Part model, mm, in its own coordinate system. A direction names the side the tool comes from. Give positions to 0.01 mm unless a question says otherwise; leave off trailing zeros. Order: outer loops, then holes, each group sorted by start corner. A loop starts at its lowest first (then second) coordinate and runs counter-clockwise, first axis right, second up. Notation, with made-up numbers: M 52.25,44.5 L 98.25,44.5 A23 cw 98.25,67.5 Z; hole C 40.25,26 d6. An arc over 180 degrees is marked long. One line per question, with ' | ' between items.
```python
from build123d import *

# Parameters (mm, degrees)
SKETCH_1_R          = 1.5
EXTRUDE_1_DEPTH     = 3.3
CUT_EXTRUDE_1_DEPTH = 3.3


with BuildPart() as part:
    # Эскиз1 → Бобышка-Вытянуть1 (new body)
    with BuildSketch(Plane(origin=(0, 0, 0), x_dir=(1, 0, 0), z_dir=(0, 1, 0))):
        Polygon((0, 0), (0, 125), (-14, 125), (-14, 14), (-68, 14), (-68, 0), align=None)
        with Locations((-30, 4)):
            Circle(SKETCH_1_R, mode=Mode.SUBTRACT)
    extrude(amount=EXTRUDE_1_DEPTH)

    # Эскиз2 → Вырез-Вытянуть1 (cut)
    with BuildSketch(Plane(origin=(0, 3.3, 0), x_dir=(1, 0, 0), z_dir=(0, 1, 0))):
        Polygon((-15.4, 14), (-14.339339828, 12.939339828), (-12.939339828, 14.339339828), (-14, 15.4), align=None)
    extrude(amount=-CUT_EXTRUDE_1_DEPTH, mode=Mode.SUBTRACT)


solid = part.part
```
1. Mould opens along Z. For faces 3 (the flat face through (-34, 2, 0)), 4 (the flat face through (-11, 3.3, -49)), 5 (the cylindrical face through (-31.5, 1.63, -4.07)) say: released by +Z, released by -Z, zero draft, split by the parting line, or undercut.
Worked out:
face 3: released by +Z | face 4: zero draft | face 5: undercut
2. Slice it at C-C on z = -4. Give the cut face in (x, y).
Worked out:
outline: M -68,0 L -31.5,0 L -31.5,3.3 L -68,3.3 Z; M -28.5,0 L 0,0 L 0,3.3 L -28.5,3.3 Z
3. Slice it at A-A on y = 1.6. Give the cut face in (x, z).
Worked out:
outline: M -68,-14 L -15.4,-14 L -14.34,-12.94 L -12.94,-14.34 L -14,-15.4 L -14,-125 L 0,-125 L 0,0 L -68,0 Z; hole C -30,-4 d3
4. Slice it at B-B on x = -30. Give the cut face in (y, z), then the cut area to 3 significant figures.
Worked out:
outline: M 0,-14 L 3.3,-14 L 3.3,-5.5 L 0,-5.5 Z; M 0,-2.5 L 3.3,-2.5 L 3.3,0 L 0,0 Z | area: 36.3 mm2
5. Slice it at D-D on z = -29.5. Give the cut face in (x, y).
Worked out:
outline: M -14,0 L 0,0 L 0,3.3 L -14,3.3 Z
6. Probe L1, parallel to X at y = 2.55, z = -4; L2, parallel to Z at x = -30, y = 1.1; L3, parallel to X at y = 1.7, z = -27. List the from-to ranges inside material, lowest first. Write a range as from..to.
Worked out:
L1: x = -68..-31.5, -28.5..0 | L2: z = -14..-5.5, -2.5..0 | L3: x = -14..0
7. Tool access for faces 1 (the flat face through (-14, 2, -71)), 2 (the flat face through (-68, 2, -7)): list every direction of +Z, -Z, +X, -X, +Y, -Y with a clear straight run to the whole face (end or side of a thin tool).
Worked out:
face 1: -Z, -X, +Y, -Y | face 2: +Z, -Z, -X, +Y, -Y
8. Drop a flat-ended pin along its axis: pin 1 (1.6 mm diameter, centred on y = 1, z = -66, fed in from -X). Give the stop position or say it passes through.
Worked out:
pin 1: stops at x = -14
